from build123d import *

# Parameters (mm, degrees)
SKETCH1_W           = 147
SKETCH1_H           = 151
BOSS_EXTRUDE1_DEPTH = 12
SKETCH2_R           = 9
SKETCH2_R_2         = 3.5
CUT_EXTRUDE1_DEPTH  = 13
SKETCH6_W           = 15
SKETCH6_H           = 151
BOSS_EXTRUDE2_DEPTH = 12
CUT_EXTRUDE3_DEPTH  = 13
SKETCH5_W           = 18.95
SKETCH5_H           = 151
CUT_EXTRUDE4_DEPTH  = 13
SKETCH7_R           = 3.2
CUT_EXTRUDE5_DEPTH  = 13


with BuildPart() as part:
    # Sketch1 → Boss-Extrude1 (new body)
    with BuildSketch(Plane(origin=(0, 0, 0), x_dir=(1, 0, 0), z_dir=(0, 1, 0))):
        Rectangle(SKETCH1_W, SKETCH1_H)
    extrude(amount=BOSS_EXTRUDE1_DEPTH)

    # Sketch2 → Cut-Extrude1 (cut, through all)
    with BuildSketch(Plane(origin=(0, 12, 0), x_dir=(1, 0, 0), z_dir=(0, 1, 0))):
        with Locations((39.8, 0)):
            Circle(SKETCH2_R)
        with Locations((20.65, -23)):
            Circle(SKETCH2_R_2)
        with Locations((40.65, -23)):
            Circle(SKETCH2_R_2)
        with Locations((40.65, 23)):
            Circle(SKETCH2_R_2)
        with Locations((20.65, 23)):
            Circle(SKETCH2_R_2)
    extrude(amount=-CUT_EXTRUDE1_DEPTH, mode=Mode.SUBTRACT)

    # Sketch6 → Boss-Extrude2 (add)
    with BuildSketch(Plane(origin=(0, 12, 0), x_dir=(1, 0, 0), z_dir=(0, 1, 0))):
        with Locations((-81, 0)):
            Rectangle(SKETCH6_W, SKETCH6_H)
    extrude(amount=-BOSS_EXTRUDE2_DEPTH)

    # Sketch4 → Cut-Extrude3 (cut, through all)
    with BuildSketch(Plane.XZ):
        with BuildLine():
            Line((-71.5, 53.5), (-81.5, 53.5))
            ThreePointArc((-81.5, 53.5), (-84, 51), (-81.5, 48.5))
            Line((-81.5, 48.5), (-71.5, 48.5))
            ThreePointArc((-71.5, 48.5), (-69, 51), (-71.5, 53.5))
        make_face()
        with BuildLine():
            Line((-71.5, 6.4), (-81.5, 6.4))
            ThreePointArc((-81.5, 6.4), (-84, 3.9), (-81.5, 1.4))
            Line((-81.5, 1.4), (-71.5, 1.4))
            ThreePointArc((-71.5, 1.4), (-69, 3.9), (-71.5, 6.4))
        make_face()
        with BuildLine():
            Line((-57.95, 47.45), (-47.95, 47.45))
            ThreePointArc((-47.95, 47.45), (-27.95, 27.45), (-47.95, 7.45))
            Line((-47.95, 7.45), (-57.95, 7.45))
            ThreePointArc((-57.95, 7.45), (-77.95, 27.45), (-57.95, 47.45))
        make_face()
        with BuildLine():
            Line((-34.4, 1.4), (-24.4, 1.4))
            ThreePointArc((-24.4, 1.4), (-21.9, 3.9), (-24.4, 6.4))
            Line((-24.4, 6.4), (-34.4, 6.4))
            ThreePointArc((-34.4, 6.4), (-36.9, 3.9), (-34.4, 1.4))
        make_face()
        with BuildLine():
            Line((-34.4, 48.5), (-24.4, 48.5))
            ThreePointArc((-24.4, 48.5), (-21.9, 51), (-24.4, 53.5))
            Line((-24.4, 53.5), (-34.4, 53.5))
            ThreePointArc((-34.4, 53.5), (-36.9, 51), (-34.4, 48.5))
        make_face()
    extrude(amount=-CUT_EXTRUDE3_DEPTH, mode=Mode.SUBTRACT)

    # Sketch5 → Cut-Extrude4 (cut, through all)
    with BuildSketch(Plane(origin=(0, 12, 0), x_dir=(1, 0, 0), z_dir=(0, 1, 0))):
        with Locations((64.025, 0)):
            Rectangle(SKETCH5_W, SKETCH5_H)
    extrude(amount=-CUT_EXTRUDE4_DEPTH, mode=Mode.SUBTRACT)

    # Sketch7 → Cut-Extrude5 (cut, through all)
    with BuildSketch(Plane(origin=(0, 12, 0), x_dir=(1, 0, 0), z_dir=(0, 1, 0))):
        with Locations((23.55, -66.5)):
            Circle(SKETCH7_R)
        with Locations((-53.45, -66.5)):
            Circle(SKETCH7_R)
        with Locations((-53.45, 66.5)):
            Circle(SKETCH7_R)
        with Locations((23.55, 66.5)):
            Circle(SKETCH7_R)
    extrude(amount=-CUT_EXTRUDE5_DEPTH, mode=Mode.SUBTRACT)


solid = part.part
For this review, take the finished solid that the model builds, in its own axes (mm). A direction names the side the tool comes from. Round coordinates to 2 decimals unless told otherwise and drop trailing zeros. Loops run counter-clockwise (first coordinate to the right, second up) from the corner with the lowest first, then second, coordinate; pieces in that order, holes last. Notation, with made-up numbers: (55, 75) - (104, 75) arc R13 cw to (104, 94) - close; hole circle Ø2 at (86.25, 57). An arc over 180 degrees is marked (long way). Put each result on its own line as item: value. Start each with the question number.
1. Consider section A-A on z = 51. State the section outline as (x, y) points, plus the area to 3 significant figures.
2. Insertion check: P1, Ø9, axis at x = 40.65, z = -23, coming from the +Y side; P2, Ø6, axis at x = 23.55, z = -66.5, coming from the -Y side. Each pin has a flat end and moves straight along its axis. Give the tip position at first contact, or say it passes through.
3. Consider section D-D on z = 23. State the section outline as (x, y) points, plus the area to 3 significant figures.
4. Consider section B-B on x = -53.45. State the section outline as (y, z) points, plus the area to 3 significant figures.
5. Consider section C-C on y = 3. State how many separate pieces and enclosed holes the cut face has, plus the area to 3 significant figures.
6. For probe 1 along X at (y, z) = (7, 66.5); probe 2 along Z at (x, y) = (40.65, 8.5); probe 3 along Z at (x, y) = (-53.45, 4.5), list the stretches that pass through material, from the lowest coordinate up. Write a range as [from, to].
7. Mouldability with a two-part tool opening along X and no side actions: class faces 1 (the flat face through (-18, 0, -1)), 2 (the cylindrical face through (25.027, 6.084, -63.661)) as +X half, -X half, draft (parallel to the pull), parting line (faces both ways), or undercut.
8. For faces 3 (the flat face through (-18, 12, -1)), 4 (the cylindrical face through (-77.945, 5.916, 27.01)), list the 3-axis set-ups (+Z, -Z, +X, -X, +Y, -Y) from which the entire face can be reached by the end or side of a thin tool; tool diameter is ignored.
Result sheet:
1. outline: (-88.5, 0) - (-84, 0) - (-84, 12) - (-88.5, 12) - close; (-69, 0) - (-36.9, 0) - (-36.9, 12) - (-69, 12) - close; (-21.9, 0) - (54.55, 0) - (54.55, 12) - (-21.9, 12) - close
1. area: 1,360 mm^2
2. P1: y = 12
2. P2: through
3. outline: (-88.5, 0) - (-77.45, 0) - (-77.45, 12) - (-88.5, 12) - close; (-28.45, 0) - (17.15, 0) - (17.15, 12) - (-28.45, 12) - close; (24.15, 0) - (37.15, 0) - (37.15, 12) - (24.15, 12) - close; (44.15, 0) - (54.55, 0) - (54.55, 12) - (44.15, 12) - close
3. area: 961 mm^2
4. outline: (0, -75.5) - (12, -75.5) - (12, -69.7) - (0, -69.7) - close; (0, -63.3) - (12, -63.3) - (12, 7.45) - (0, 7.45) - close; (0, 47.45) - (12, 47.45) - (12, 63.3) - (0, 63.3) - close; (0, 69.7) - (12, 69.7) - (12, 75.5) - (0, 75.5) - close
4. area: 1,180 mm^2
5. separate pieces: 1
5. enclosed holes: 14
5. area: 19,100 mm^2
6. probe 1: [-88.5, -56.65], [-50.25, 20.35], [26.75, 54.55]
6. probe 2: [-75.5, -26.5], [-19.5, -8.96], [8.96, 19.5], [26.5, 75.5]
6. probe 3: [-75.5, -69.7], [-63.3, 7.45], [47.45, 63.3], [69.7, 75.5]
7. face 1: draft
7. face 2: undercut
8. face 3: +Z, -Z, +X, -X, +Y
8. face 4: +Y, -Y
